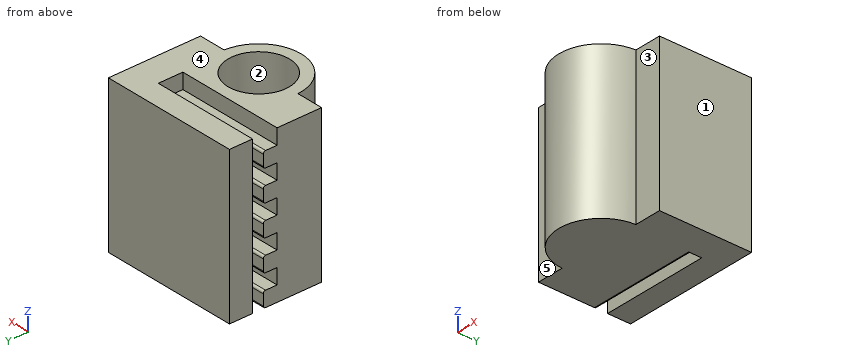
from build123d import *

# Parameters (mm, degrees)
SKETCH1_W           = 9
SKETCH1_H           = 6
BOSS_EXTRUDE1_DEPTH = 10
CUT_EXTRUDE1_START  = -2
SKETCH2_W           = 10
SKETCH2_H           = 1.6
CUT_EXTRUDE1_DEPTH  = 7
SKETCH3_R           = 2.75
BOSS_EXTRUDE2_DEPTH = 10
SKETCH4_R           = 2
CUT_EXTRUDE2_DEPTH  = 4
BOSS_EXTRUDE3_REACH = 16.573


with BuildPart() as part:
    # Sketch1 → Boss-Extrude1 (new body)
    with BuildSketch(Plane.XY):
        Rectangle(SKETCH1_W, SKETCH1_H)
    extrude(amount=BOSS_EXTRUDE1_DEPTH)

    # Sketch2 → Cut-Extrude1 (cut)
    with BuildSketch(Plane(origin=(4.5, 0, 0), x_dir=(0, 0, -1), z_dir=(1, 0, 0)).offset(CUT_EXTRUDE1_START)):
        with Locations((-5, 0.7)):
            Rectangle(SKETCH2_W, SKETCH2_H)
    extrude(amount=-CUT_EXTRUDE1_DEPTH, mode=Mode.SUBTRACT)

    # Sketch3 → Boss-Extrude2 (add, through all)
    with BuildSketch(Plane.XY.offset(10)):
        with Locations((0, -2.85)):
            Circle(SKETCH3_R)
    extrude(amount=-BOSS_EXTRUDE2_DEPTH)

    # Sketch4 → Cut-Extrude2 (cut)
    with BuildSketch(Plane.XY.offset(10)):
        with Locations((0, -2.85)):
            Circle(SKETCH4_R)
    extrude(amount=-CUT_EXTRUDE2_DEPTH, mode=Mode.SUBTRACT)

    # Sketch5 → Boss-Extrude3 (add, up to next)
    with BuildSketch(Plane.ZY.offset(4.5), mode=Mode.PRIVATE) as boss_extrude3_sk1:
        with BuildLine():
            Line((0, -0.1), (1, -0.1))
            Line((1, -0.1), (1, 0.65))
            ThreePointArc((1, 0.65), (0.956066017, 0.756066017), (0.85, 0.8))
            Line((0.85, 0.8), (0.15, 0.8))
            ThreePointArc((0.15, 0.8), (0.043933983, 0.756066017), (0, 0.65))
            Line((0, 0.65), (0, -0.1))
        make_face()
    boss_extrude3_tool1 = extrude(boss_extrude3_sk1.sketch, amount=-BOSS_EXTRUDE3_REACH, mode=Mode.PRIVATE) - part.part
    # Sketch5 → Boss-Extrude3 (add, up to next)
    with BuildSketch(Plane.ZY.offset(4.5), mode=Mode.PRIVATE) as boss_extrude3_sk2:
        with BuildLine():
            Line((2, -0.1), (2, 0.65))
            ThreePointArc((2, 0.65), (2.043933983, 0.756066017), (2.15, 0.8))
            Line((2.15, 0.8), (2.85, 0.8))
            ThreePointArc((2.85, 0.8), (2.956066017, 0.756066017), (3, 0.65))
            Line((3, 0.65), (3, -0.1))
            Line((3, -0.1), (2, -0.1))
        make_face()
    boss_extrude3_tool2 = extrude(boss_extrude3_sk2.sketch, amount=-BOSS_EXTRUDE3_REACH, mode=Mode.PRIVATE) - part.part
    # Sketch5 → Boss-Extrude3 (add, up to next)
    with BuildSketch(Plane.ZY.offset(4.5), mode=Mode.PRIVATE) as boss_extrude3_sk3:
        with BuildLine():
            Line((4, -0.1), (4, 0.65))
            ThreePointArc((4, 0.65), (4.043933983, 0.756066017), (4.15, 0.8))
            Line((4.15, 0.8), (4.85, 0.8))
            ThreePointArc((4.85, 0.8), (4.956066017, 0.756066017), (5, 0.65))
            Line((5, 0.65), (5, -0.1))
            Line((5, -0.1), (4, -0.1))
        make_face()
    boss_extrude3_tool3 = extrude(boss_extrude3_sk3.sketch, amount=-BOSS_EXTRUDE3_REACH, mode=Mode.PRIVATE) - part.part
    # Sketch5 → Boss-Extrude3 (add, up to next)
    with BuildSketch(Plane.ZY.offset(4.5), mode=Mode.PRIVATE) as boss_extrude3_sk4:
        with BuildLine():
            Line((6, -0.1), (6, 0.65))
            ThreePointArc((6, 0.65), (6.043933983, 0.756066017), (6.15, 0.8))
            Line((6.15, 0.8), (6.85, 0.8))
            ThreePointArc((6.85, 0.8), (6.956066017, 0.756066017), (7, 0.65))
            Line((7, 0.65), (7, -0.1))
            Line((7, -0.1), (6, -0.1))
        make_face()
    boss_extrude3_tool4 = extrude(boss_extrude3_sk4.sketch, amount=-BOSS_EXTRUDE3_REACH, mode=Mode.PRIVATE) - part.part
    # Sketch5 → Boss-Extrude3 (add, up to next)
    with BuildSketch(Plane.ZY.offset(4.5), mode=Mode.PRIVATE) as boss_extrude3_sk5:
        with BuildLine():
            Line((8, -0.1), (8, 0.65))
            ThreePointArc((8, 0.65), (8.043933983, 0.756066017), (8.15, 0.8))
            Line((8.15, 0.8), (8.85, 0.8))
            ThreePointArc((8.85, 0.8), (8.956066017, 0.756066017), (9, 0.65))
            Line((9, 0.65), (9, -0.1))
            Line((9, -0.1), (8, -0.1))
        make_face()
    boss_extrude3_tool5 = extrude(boss_extrude3_sk5.sketch, amount=-BOSS_EXTRUDE3_REACH, mode=Mode.PRIVATE) - part.part
    add(boss_extrude3_tool1.solids().sort_by_distance((-4.5, 0.345482, 0.5))[0])
    add(boss_extrude3_tool2.solids().sort_by_distance((-4.5, 0.345482, 2.5))[0])
    add(boss_extrude3_tool3.solids().sort_by_distance((-4.5, 0.345482, 4.5))[0])
    add(boss_extrude3_tool4.solids().sort_by_distance((-4.5, 0.345482, 6.5))[0])
    add(boss_extrude3_tool5.solids().sort_by_distance((-4.5, 0.345482, 8.5))[0])


solid = part.part
Model file for the job. Use its own axes, mm. Face numbers are marked on the shaded views. A direction names the side the tool comes from. Give positions to 0.01 mm unless a question says otherwise; leave off trailing zeros. Write each loop counter-clockwise with the first axis right and the second up, starting at its lowest first coordinate (ties: lowest second). Pieces come first, ordered by that corner, then holes. Notation, with made-up numbers: (30, 50) -> (86, 50) arc R36 ccw to (86, 84) -> close; hole circle Ø11 at (8.5, 51). An arc over 180 degrees is marked (long way). Write item = value, one per line.
(1) Mould opens along Y. For the marked faces 1, 2 and 3 say: released by +Y, released by -Y, zero draft, split by the parting line, or undercut.
Determined:
face_1 = zero draft
face_2 = undercut
face_3 = released by -Y
(2) Slice it at B-B, the plane y = -2.85. Give the cut face in (x, z).
Determined:
outline = (-4.5, 0) -> (4.5, 0) -> (4.5, 10) -> (2, 10) -> (2, 6) -> (-2, 6) -> (-2, 10) -> (-4.5, 10) -> close
(3) Probe line 1 along Y through (x, z) = (0, 8.65); line 2 along Y through (x, z) = (0, 9.15); line 3 along Y through (x, z) = (-3.25, 3.5). List the from-to ranges inside material, lowest first.
Determined:
line_1 = -5.6 to -4.85, -0.85 to 0.8, 1.5 to 3
line_2 = -5.6 to -4.85, -0.85 to -0.1, 1.5 to 3
line_3 = -3 to -0.1, 1.5 to 3
(4) Slice it at C-C, the plane x = 3.25. Give the cut face in (y, z).
Determined:
outline = (-3, 0) -> (3, 0) -> (3, 10) -> (-3, 10) -> close
(5) Slice it at D-D, the plane y = 0.5. Give the cut face in (x, z).
Determined:
outline = (-4.5, 0) -> (4.5, 0) -> (4.5, 10) -> (2.5, 10) -> (2.5, 9) -> (-4.5, 9) -> (-4.5, 8) -> (2.5, 8) -> (2.5, 7) -> (-4.5, 7) -> (-4.5, 6) -> (2.5, 6) -> (2.5, 5) -> (-4.5, 5) -> (-4.5, 4) -> (2.5, 4) -> (2.5, 3) -> (-4.5, 3) -> (-4.5, 2) -> (2.5, 2) -> (2.5, 1) -> (-4.5, 1) -> close
(6) Flat gauge pins, fed straight in: P1, Ø3, axis at x = 3.5, z = 2, coming from the -Y side; P2, Ø4, axis at x = -1, y = -4.5, coming from the +Z side; P3, Ø1.4, axis at x = 3.5, z = 7, coming from the -Y side; P4, Ø5, axis at x = 3, z = 7, coming from the -Y side. Where does each tip first touch, or does it go through?
Determined:
P1 = -4.74
P2 = 10
P3 = -3
P4 = -5.55
(7) Tool access for the marked faces 4 and 5: list every direction of +Z, -Z, +X, -X, +Y, -Y with a clear straight run to the whole face (end or side of a thin tool).
Determined:
face_4 = +Z, +X, -X, +Y, -Y
face_5 = +Z, -Z, -X, -Y
